Can you work these out from the model? Positions are in its coordinate system, mm. Face numbers are marked on the shaded views. Coordinates: 2 decimals unless noted, no trailing zeros. Order: outer loops, then holes, each group sorted by start corner. A loop starts at its lowest first (then second) coordinate and runs counter-clockwise, first axis right, second up. Notation, with made-up numbers: (-36, 60.5) - (-19, 60.5) arc R17 ccw to (-19, 91.5) - close; hole circle Ø8 at (-1.75, 10.25). An arc over 180 degrees is marked (long way). Use a Markdown table: item, result. Add a question column.
(1) I want a section at D-D (z = 0). List the corners of the cut face in (x, y) for me, and give its area (3 significant figures).
(2) We'd pull the mould along X, two halves only. Please class the marked faces 1, 2 and 3: pulls with the +X half, pulls with the -X half, needs draft (parallel to the pull), parting line crosses it, or undercut.
(3) I want a section at A-A (x = 0). List the corners of the cut face in (y, z) for me.
(4) If I drill on L1, parallel to Z at x = 0, y = 0.3; L2, parallel to X at y = -0.05, z = 0; L3, parallel to Z at x = -0.35, y = -1.25, over which ranges is the centre line in solid material (lowest first)? Write a range as [from, to].
(5) I want a section at C-C (z = 7). List the corners of the cut face in (x, y) for me, and give its area (3 significant figures).
(6) I want a section at B-B (y = 0). List the corners of the cut face in (x, z) for me, and give its area (3 significant figures).
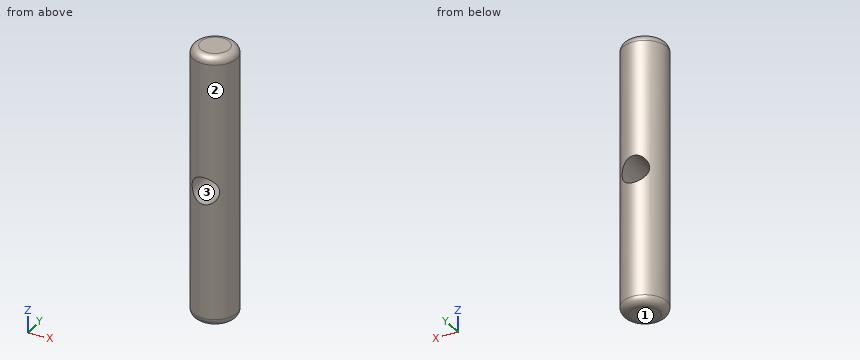
```python
from build123d import *

# Parameters (mm, degrees)
F0_R     = 1.45
F1_DEPTH = 9
F2_R     = 0.9
F3_DEPTH = 12.5
F4_R     = 0.5


with BuildPart() as f1:
    # F0 (on Top) → F1 (new body, symmetric)
    with BuildSketch(Plane.XY):
        Circle(F0_R)
    extrude(amount=F1_DEPTH, both=True)

    # F2 (on Front) → F3 (cut, symmetric)
    with BuildSketch(Plane.XZ):
        Circle(F2_R)
    extrude(amount=F3_DEPTH, both=True, mode=Mode.SUBTRACT)

    # F4
    f4_edges = [f1.edges().sort_by_distance(p)[0] for p in [
        (-1.45, 0, 9),
        (-1.45, 0, -9),
    ]]
    fillet(f4_edges, radius=F4_R)


solid = f1.part
```
Answers follow:
| question | item | result |
|---|---|---|
| 1 | outline | (-0.9, -1.14) - (-0.9, 1.14) arc R1.45 ccw to start; (0.9, -1.14) arc R1.45 ccw to (0.9, 1.14) - close |
| 1 | area | 1.74 mm² |
| 2 | face 1 | needs draft |
| 2 | face 2 | parting line crosses it |
| 2 | face 3 | undercut |
| 3 | outline | (-1.45, -8.5) arc R0.5 ccw to (-0.95, -9) - (0.95, -9) arc R0.5 ccw to (1.45, -8.5) - (1.45, -0.9) - (-1.45, -0.9) - close; (-1.45, 0.9) - (1.45, 0.9) - (1.45, 8.5) arc R0.5 ccw to (0.95, 9) - (-0.95, 9) arc R0.5 ccw to (-1.45, 8.5) - close |
| 4 | L1 | z = [-9, -0.9], [0.9, 9] |
| 4 | L2 | x = [-1.45, -0.9], [0.9, 1.45] |
| 4 | L3 | z = [-8.86, -0.83], [0.83, 8.86] |
| 5 | outline | circle Ø2.9 at (0, 0) |
| 5 | area | 6.61 mm² |
| 6 | outline | (-1.45, -8.5) arc R0.5 ccw to (-0.95, -9) - (0.95, -9) arc R0.5 ccw to (1.45, -8.5) - (1.45, 8.5) arc R0.5 ccw to (0.95, 9) - (-0.95, 9) arc R0.5 ccw to (-1.45, 8.5) - close; hole circle Ø1.8 at (0, 0) |
| 6 | area | 49.4 mm² |
